Input: part model. Units: mm. Frame: model coordinates. Give positions to 0.01 mm unless a question says otherwise; leave off trailing zeros. Order: outer loops, then holes, each group sorted by start corner. A loop starts at its lowest first (then second) coordinate and runs counter-clockwise, first axis right, second up. Notation, with made-up numbers: M 30.5,52.25 L 81.5,52.25 A15 ccw 81.5,56.25 Z; hole C -23.75,46.5 d8. An arc over 180 degrees is marked long. Use a Markdown table: item, result.
from build123d import *

# Parameters (mm, degrees)
F0_W     = 320
F0_H     = 320
F0_R     = 115.5
F1_DEPTH = 19.05


with BuildPart() as f1:
    # F0 (on Front) → F1 (new body)
    with BuildSketch(Plane.XZ):
        Rectangle(F0_W, F0_H)
        Circle(F0_R, mode=Mode.SUBTRACT)
    extrude(amount=-F1_DEPTH)


solid = f1.part
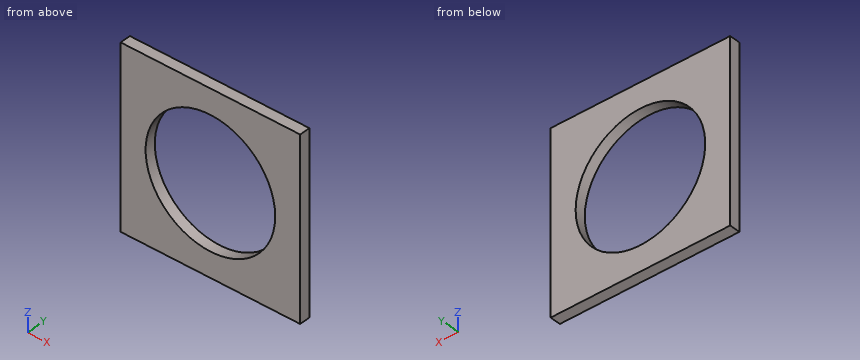
1) Material intervals for line 1 (Z direction, x = 0, y = 9.25); line 2 (Z direction, x = -27, y = 3.75); line 3 (X direction, y = 7, z = -106), sorted ascending. Write a range as from..to.
Response values:
| item | result |
|---|---|
| line 1 | z = -160..-115.5, 115.5..160 |
| line 2 | z = -160..-112.3, 112.3..160 |
| line 3 | x = -160..-45.87, 45.87..160 |
2) Cut plane C-C on y = 10. Return loops of the section in (x, z), and give its area (3 significant figures).
Response values:
| item | result |
|---|---|
| outline | M -160,-160 L 160,-160 L 160,160 L -160,160 Z; hole C 0,0 d231 |
| area | 60,500 mm² |
3) Cut plane A-A on x = 0. Return loops of the section in (y, z).
Response values:
| item | result |
|---|---|
| outline | M 0,-160 L 19.05,-160 L 19.05,-115.5 L 0,-115.5 Z; M 0,115.5 L 19.05,115.5 L 19.05,160 L 0,160 Z |
4) Cut plane B-B on z = 0. Return loops of the section in (x, y).
Response values:
| item | result |
|---|---|
| outline | M -160,0 L -115.5,0 L -115.5,19.05 L -160,19.05 Z; M 115.5,0 L 160,0 L 160,19.05 L 115.5,19.05 Z |
